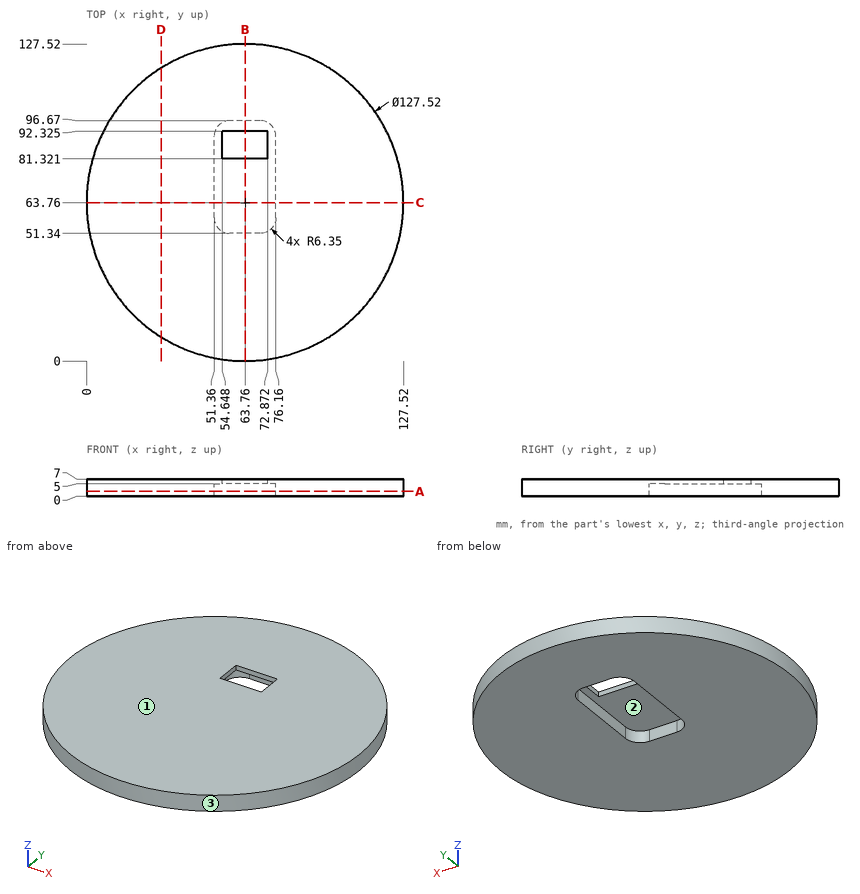
Job drawing, mm, ordinate dimensions from the low corner. One solid piece. Give positions to 0.01 mm unless a question says otherwise; leave off trailing zeros. Write each loop counter-clockwise with the first axis right and the second up, starting at its lowest first coordinate (ties: lowest second). Pieces come first, ordered by that corner, then holes. Notation, with made-up numbers: (17.25, 27.25) - (52.25, 27.25) arc R12 cw to (52.25, 45.25) - close; hole circle Ø7 at (14, -14). An arc over 180 degrees is marked (long way). Answer as CSV lines item,"result".
1. Band-saw the part on D-D (x = 30). Write the cut outline in (y, z), and give its area (3 significant figures).
Responses:
outline,"(9.67, 0) - (117.85, 0) - (117.85, 7) - (9.67, 7) - close"
area,"757 mm2"
2. Band-saw the part on A-A (z = 2). Write the cut outline in (x, y), and give its area (3 significant figures).
Responses:
outline,"circle Ø127.52 at (63.76, 63.76); hole (51.36, 57.69) arc R6.35 ccw to (57.71, 51.34) - (69.81, 51.34) arc R6.35 ccw to (76.16, 57.69) - (76.16, 90.32) arc R6.35 ccw to (69.81, 96.67) - (57.71, 96.67) arc R6.35 ccw to (51.36, 90.32) - close"
area,"11,700 mm2"
3. Pin check, flat tips, straight feed: pin 1 (1 mm diameter, centred on x = 35, z = 5.5, fed in from +Y) (1 decimal); pin 2 (4 mm diameter, centred on y = 72.5, z = 2, fed in from +X); pin 3 (1 mm diameter, centred on x = 63, z = 6.5, fed in from +Y); pin 4 (1.5 mm diameter, centred on x = 104, y = 29, fed in from -Z). Stop position of each tip, or through.
Responses:
pin 1,"stops at y = 120.9"
pin 2,"stops at x = 127.16"
pin 3,"stops at y = 127.52"
pin 4,"stops at z = 0"
4. Band-saw the part on C-C (y = 63.76). Write the cut outline in (x, z).
Responses:
outline,"(0, 0) - (51.36, 0) - (51.36, 5) - (76.16, 5) - (76.16, 0) - (127.52, 0) - (127.52, 7) - (0, 7) - close"
5. Two-plate mould, pull along Y, no slides. Class the marked faces 1, 2 and 3: +Y half, -Y half, draft (parallel to the pull), parting line (faces both ways), or undercut.
Responses:
face 1,"draft"
face 2,"undercut"
face 3,"parting line"
6. Drill centre lines: L1, parallel to Y at x = 61, z = 4.25; L2, parallel to Y at x = 62, z = 0.75 (1 decimal); L3, parallel to X at y = 78.5, z = 1.5. Where is each one in solid material? Low to high. Write a range as [from, to].
Responses:
L1,"y = [0.06, 51.34], [96.67, 127.46]"
L2,"y = [0, 51.3], [96.7, 127.5]"
L3,"x = [1.73, 51.36], [76.16, 125.79]"
7. Band-saw the part on B-B (x = 63.76). Write the cut outline in (y, z) (1 decimal), and give its area (3 significant figures).
Responses:
outline,"(0, 0) - (51.3, 0) - (51.3, 5) - (81.3, 5) - (81.3, 7) - (0, 7) - close; (92.3, 5) - (96.7, 5) - (96.7, 0) - (127.5, 0) - (127.5, 7) - (92.3, 7) - close"
area,"644 mm2"
